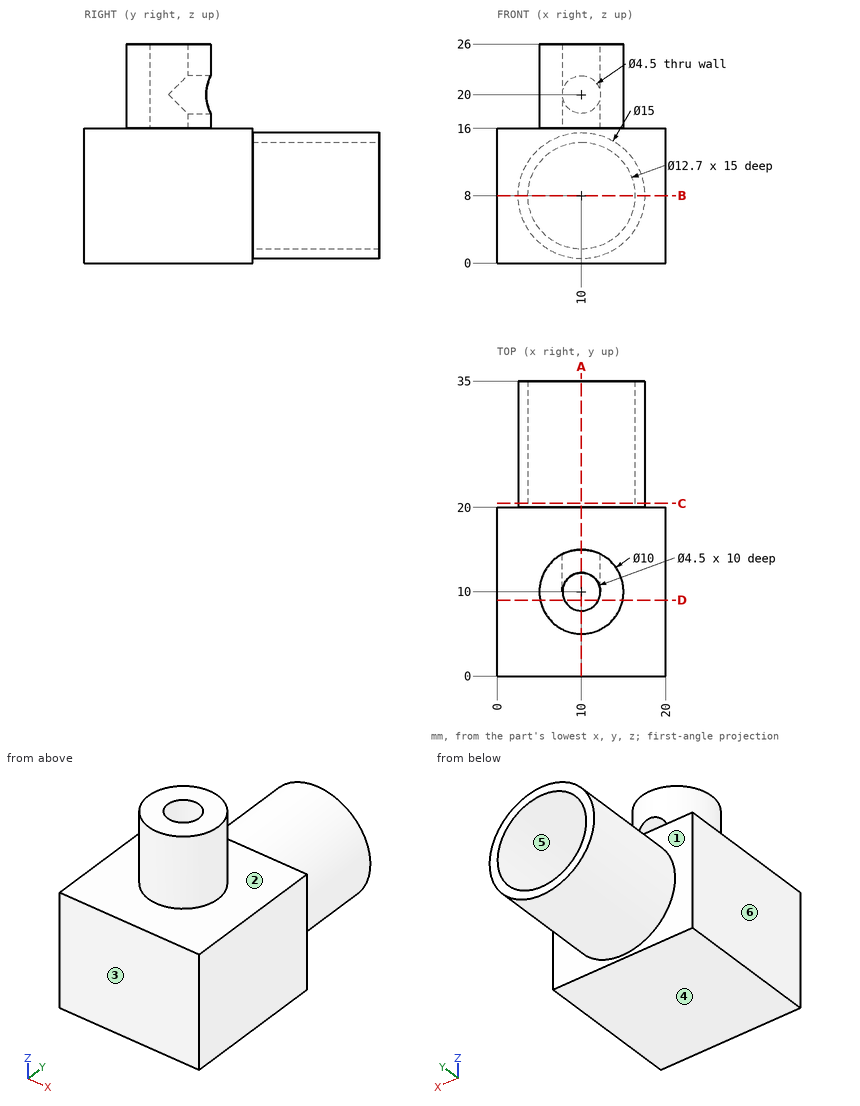
Verification items for this drawing (mm, ordinates from the low corner). A direction names the side the tool comes from. Give positions to 0.01 mm unless a question says otherwise; leave off trailing zeros. Write each loop counter-clockwise with the first axis right and the second up, starting at its lowest first coordinate (ties: lowest second). Pieces come first, ordered by that corner, then holes.
1) Material ranges on L1, parallel to X at y = 29, z = 8; L2, parallel to Z at x = 9.75, y = 24; L3, parallel to Z at x = 10, y = 11.55, recorded low to high.
2) Access from +Z, -Z, +X, -X, +Y, -Y to the whole of each face (thin tool, end or side, straight path). Record for the marked faces 1, 2 and 3.
3) Release check for a two-part mould opening along X. For the marked faces 4, 5 and 6 record: pulls with the +X half, pulls with the -X half, needs draft (parallel to the pull), parting line crosses it, or undercut.
4) Section check B-B, the plane z = 8. Record the boundary of the cut face in (x, y), and give its area (4 significant figures).
5) Gauge pin test, flat ends, axial feed: pin 1 (1.5 mm diameter, centred on x = 7.5, y = 23, fed in from -Z); pin 2 (3 mm diameter, centred on x = 3.5, y = 20.5, fed in from +Z); pin 3 (1.5 mm diameter, centred on x = 16.5, y = 21.5, fed in from -Z). Record the tip position at first contact, or that the pin passes through.
6) Section check C-C, the plane y = 20.5. Record the boundary of the cut face in (x, z).
7) Section check D-D, the plane y = 9. Record the boundary of the cut face in (x, z), and give its area (3 significant figures).
8) Section check A-A, the plane x = 10. Record the boundary of the cut face in (y, z).
Computed:
1. L1: x = 2.5 to 3.65, 16.35 to 17.5
1. L2: z = 0.5 to 1.65, 14.35 to 15.5
1. L3: z = 0 to 16
2. face 1: +Y
2. face 2: +Z
2. face 3: +Z, -Z, +X, -X, -Y
3. face 4: needs draft
3. face 5: undercut
3. face 6: pulls with the -X half
4. outline: (0, 0) - (20, 0) - (20, 20) - (17.5, 20) - (17.5, 35) - (16.35, 35) - (16.35, 20) - (3.65, 20) - (3.65, 35) - (2.5, 35) - (2.5, 20) - (0, 20) - close
4. area: 434.5 mm2
5. pin 1: stops at z = 0.71
5. pin 2: stops at z = 16
5. pin 3: stops at z = 3.18
6. outline: circle Ø15 at (10, 8); hole circle Ø12.7 at (10, 8)
7. outline: (0, 0) - (20, 0) - (20, 16) - (14.9, 16) - (14.9, 26) - (12.02, 26) - (12.02, 16) - (7.98, 16) - (7.98, 26) - (5.1, 26) - (5.1, 16) - (0, 16) - close
7. area: 378 mm2
8. outline: (0, 0) - (20, 0) - (20, 0.5) - (35, 0.5) - (35, 1.65) - (20, 1.65) - (20, 14.35) - (35, 14.35) - (35, 15.5) - (20, 15.5) - (20, 16) - (15, 16) - (15, 17.75) - (12.25, 17.75) - (12.25, 16) - (7.75, 16) - (7.75, 26) - (5, 26) - (5, 16) - (0, 16) - close; (12.25, 22.25) - (15, 22.25) - (15, 26) - (12.25, 26) - close
